```python
from build123d import *

# Parameters (mm, degrees)
SKETCH_1_R          = 4.6
EXTRUDE_1_DEPTH     = 4
EXTRUDE_START       = -4
SKETCH_1_4_R        = 4.6
SKETCH_1_4_W        = 4
SKETCH_1_4_H        = 50.693747285
EXTRUDE_2_DEPTH     = 4
EXTRUDE_3_DEPTH     = 12
SKETCH_4_R          = 2.2
CUT_EXTRUDE_2_DEPTH = 12
SKETCH_4_3_R        = 1.6
CUT_EXTRUDE_3_DEPTH = 64.691687079
RIB_6_REACH         = 53.839
SKETCH_6_WALL_W     = 120.90928936
SKETCH_6_WALL_H     = 5
RIB_7_REACH         = 51.729
SKETCH_8_WALL_W     = 116.68872775
SKETCH_8_WALL_H     = 5


with BuildPart() as part:
    # 草图1 → 凸台-拉伸1 (new body)
    with BuildSketch(Plane.XY):
        with BuildLine():
            ThreePointArc((20.5, 46.874119675), (20.438884601, 46.271660298), (20.258028466, 45.693747285))
            Line((20.258028466, 45.693747285), (4, 45.693747285))
            Line((4, 45.693747285), (4, 52.693747285))
            Line((4, 52.693747285), (0, 52.693747285))
            Line((0, 52.693747285), (0, 2))
            Line((0, 2), (4, 2))
            Line((4, 2), (4, 9))
            Line((4, 9), (23.999999933, 9))
            ThreePointArc((23.999999933, 9), (33.430862955, 13.579836665), (35.663090571, 23.823529412))
            Line((35.663090571, 23.823529412), (31.775393714, 39.882352941))
            ThreePointArc((31.775393714, 39.882352941), (30.656120461, 42.438024382), (28.727272727, 44.453905218))
            ThreePointArc((28.727272727, 44.453905218), (28.15133251, 45.007636077), (27.741971534, 45.693747285))
            ThreePointArc((27.741971534, 45.693747285), (27.561115399, 46.271660298), (27.5, 46.874119675))
            Line((27.5, 46.874119675), (27.5, 52.693747285))
            Line((27.5, 52.693747285), (24.5, 52.693747285))
            Line((24.5, 52.693747285), (24.5, 42.220485754))
            ThreePointArc((24.5, 42.220485754), (24, 33.75), (23.5, 42.220485754))
            Line((23.5, 42.220485754), (23.5, 52.693747285))
            Line((23.5, 52.693747285), (20.5, 52.693747285))
            Line((20.5, 52.693747285), (20.5, 46.874119675))
        make_face()
        with Locations((24, 21)):
            Circle(SKETCH_1_R, mode=Mode.SUBTRACT)
    extrude(amount=EXTRUDE_1_DEPTH)

    # 草图1<4> → 凸台-拉伸2 (add)
    # profile 1 of 2: a face of its own
    with BuildSketch(Plane.XY.offset(EXTRUDE_START)):
        with BuildLine():
            ThreePointArc((19.272727273, 44.453905218), (17.343879539, 42.438024382), (16.224606286, 39.882352941))
            Line((16.224606286, 39.882352941), (12.336909429, 23.823529412))
            ThreePointArc((12.336909429, 23.823529412), (24, 9), (35.663090571, 23.823529412))
            Line((35.663090571, 23.823529412), (31.775393714, 39.882352941))
            ThreePointArc((31.775393714, 39.882352941), (30.656120461, 42.438024382), (28.727272727, 44.453905218))
            ThreePointArc((28.727272727, 44.453905218), (28.15133251, 45.007636077), (27.741971534, 45.693747285))
            ThreePointArc((27.741971534, 45.693747285), (27.561115399, 46.271660298), (27.5, 46.874119675))
            Line((27.5, 46.874119675), (27.5, 52.693747285))
            Line((27.5, 52.693747285), (24.5, 52.693747285))
            Line((24.5, 52.693747285), (24.5, 42.220485754))
            ThreePointArc((24.5, 42.220485754), (24, 33.75), (23.5, 42.220485754))
            Line((23.5, 42.220485754), (23.5, 52.693747285))
            Line((23.5, 52.693747285), (20.5, 52.693747285))
            Line((20.5, 52.693747285), (20.5, 46.874119675))
            ThreePointArc((20.5, 46.874119675), (20.438884601, 46.271660298), (20.258028466, 45.693747285))
            ThreePointArc((20.258028466, 45.693747285), (19.84866749, 45.007636077), (19.272727273, 44.453905218))
        make_face()
        with Locations((24, 21)):
            Circle(SKETCH_1_4_R, mode=Mode.SUBTRACT)
    # profile 2 of 2: a face of its own
    with BuildSketch(Plane.XY.offset(EXTRUDE_START)):
        with Locations((2, 27.346873643)):
            Rectangle(SKETCH_1_4_W, SKETCH_1_4_H)
    extrude(amount=EXTRUDE_2_DEPTH)

    # 草图1<5> → 凸台-拉伸3 (add)
    with BuildSketch(Plane.XY.offset(EXTRUDE_START)):
        Polygon((4, 45.693747285), (4, 9), (4, 2), (0, 2), (0, 52.693747285), (4, 52.693747285), align=None)
    extrude(amount=-EXTRUDE_3_DEPTH)

    # 草图4 → 切除-拉伸2 (cut)
    with BuildSketch(Plane(origin=(4, 0, 0), x_dir=(0, 0, -1), z_dir=(1, 0, 0))):
        with Locations(Location((6, 48.693747285, 0), (0, 0, 90))):
            Circle(SKETCH_4_R)
        with Locations(Location((6, 6, 0), (0, 0, 90))):
            Circle(SKETCH_4_R)
    extrude(amount=-CUT_EXTRUDE_2_DEPTH, mode=Mode.SUBTRACT)

    # 草图4<3> → 切除-拉伸3 (cut, through all)
    with BuildSketch(Plane(origin=(4, 0, 0), x_dir=(0, 0, -1), z_dir=(1, 0, 0))):
        with Locations((0, 49.693747285)):
            Circle(SKETCH_4_3_R)
    extrude(amount=CUT_EXTRUDE_3_DEPTH, mode=Mode.SUBTRACT)

    # 草图6 wall → 筋6 (add, up to next)
    with BuildSketch(Plane(origin=(7, 19, -7), x_dir=(0.393919298579, 0, 0.919145030018), z_dir=(-0.919145030018, 0, 0.393919298579)), mode=Mode.PRIVATE) as rib_6_sk1:
        Rectangle(SKETCH_6_WALL_W, SKETCH_6_WALL_H)
    rib_6_tool1 = extrude(rib_6_sk1.sketch, amount=RIB_6_REACH, mode=Mode.PRIVATE) - part.part
    add(rib_6_tool1.solids().sort_by_distance((7, 19, -7))[0])

    # 草图8 wall → 筋7 (add, up to next)
    with BuildSketch(Plane(origin=(7, 32.346873642, -7), x_dir=(0.393919298579, 0, 0.919145030018), z_dir=(-0.919145030018, 0, 0.393919298579)), mode=Mode.PRIVATE) as rib_7_sk1:
        Rectangle(SKETCH_8_WALL_W, SKETCH_8_WALL_H)
    rib_7_tool1 = extrude(rib_7_sk1.sketch, amount=RIB_7_REACH, mode=Mode.PRIVATE) - part.part
    add(rib_7_tool1.solids().sort_by_distance((7, 32.346873642, -7))[0])


solid = part.part
```
Model file for the job. Use its own axes, mm. A direction names the side the tool comes from. Coordinates: 2 decimals unless noted, no trailing zeros. Order: outer loops, then holes, each group sorted by start corner. A loop starts at its lowest first (then second) coordinate and runs counter-clockwise, first axis right, second up. Notation, with made-up numbers: (4.25, 30.5) - (42.25, 30.5) arc R13 cw to (42.25, 37.5) - close; hole circle Ø11 at (3, 77). An arc over 180 degrees is marked (long way). Return JSON: item names as keys, results as strings. Group by question number.
1) Flat gauge pins, fed straight in: P1, Ø2.5, axis at y = 49.69, z = 0, coming from the +X side; P2, Ø4, axis at y = 49.69, z = 0, coming from the +X side; P3, Ø10.5, axis at x = 24, y = 21, coming from the -Z side; P4, Ø1.8, axis at x = 8, z = -10, coming from the +Y side. Where does each tip first touch, or does it go through?
2) Mould opens along X. For faces 1 (the flat face through (0, 27, -6)), 2 (the flat face through (23.5, 47, 0)), 3 (the flat face through (14, 9, 2)), 4 (the flat face through (6, 16.5, -5)) say: released by +X, released by -X, zero draft, split by the parting line, or undercut.
3) Probe line 1 (X direction, y = 49.5, z = 3.25); line 2 (X direction, y = 38, z = -2); line 3 (Z direction, x = 21, y = 31). List the from-to ranges inside material, lowest first. Write a range as from..to.
4) Saw through at B-B, the plane z = -7. Write the cut outline in (x, y), plus the area to 3 significant figures.
5) Tool access for faces 5 (the cylindrical face through (21.979, 48.274, -0.738)), 6 (the flat face through (12, 45.694, 2)), 7 (the flat face through (6, 29.847, -5)), 8 (the flat face through (7, 32, -7)): list every direction of +Z, -Z, +X, -X, +Y, -Y with a clear straight run to the whole face (end or side of a thin tool).
6) Saw through at A-A, the plane y = 6. Write the cut outline in (x, z).
7) Saw through at C-C, the plane z = -9.5. Write the cut outline in (x, y).
8) Saw through at D-D, the plane x = 17. Write the cut outline in (y, z), plus the area to 3 significant figures.
Values found:
{
 "1": {"P1": "stops at x = 4", "P2": "stops at x = 27.5", "P3": "stops at z = -4", "P4": "passes through"},
 "2": {"face 1": "released by -X", "face 2": "undercut", "face 3": "zero draft", "face 4": "undercut"},
 "3": {"line 1": "x = 0..4, 20.5..23.5, 24.5..27.5", "line 2": "x = 0..4, 15.77..19.75, 28.25..32.23", "line 3": "z = -4..4"},
 "4": {"outline": "(0, 2) - (4, 2) - (4, 4.04) - (0, 4.04) - close; (0, 7.96) - (4, 7.96) - (4, 16.5) - (7, 16.5) - (7, 21.5) - (4, 21.5) - (4, 29.85) - (7, 29.85) - (7, 34.85) - (4, 34.85) - (4, 46.73) - (0, 46.73) - close; (0, 50.65) - (4, 50.65) - (4, 52.69) - (0, 52.69) - close", "area": "201 mm²"},
 "5": {"face 5": "+X", "face 6": "+Z, -Z, +Y", "face 7": "-Z", "face 8": "-Z, +Y, -Y"},
 "6": {"outline": "(0, -16) - (4, -16) - (4, -8.2) - (0, -8.2) - close; (0, -3.8) - (4, -3.8) - (4, 4) - (0, 4) - close"},
 "7": {"outline": "(0, 2) - (4, 2) - (4, 16.5) - (5.93, 16.5) - (5.93, 21.5) - (4, 21.5) - (4, 29.85) - (5.93, 29.85) - (5.93, 34.85) - (4, 34.85) - (4, 52.69) - (0, 52.69) - close"},
 "8": {"outline": "(9, 0) - (11.25, 0) - (11.25, -4) - (41.87, -4) - (41.87, 0) - (45.69, 0) - (45.69, 4) - (9, 4) - close", "area": "269 mm²"}
}
